Could you check a few things on this model? Use its own coordinates, in mm. Face numbers are marked on the shaded views. A direction names the side the tool comes from. Coordinates: 2 decimals unless noted, no trailing zeros. Write each loop counter-clockwise with the first axis right and the second up, starting at its lowest first coordinate (ties: lowest second). Pieces come first, ordered by that corner, then holes.
Autodesk Inventor part; units mm, degrees
ref_plane "Plano de trabajo1" through (15, 0, 0) normal (1, 0, 0) x (0, 1, 0)
ref_plane "Plano de trabajo2" through (0, 0, 7.5) normal (0, 0, 1) x (1, 0, 0)
ref_plane "XZ Plane" through (0, 0, 0) normal (0, 1, 0) x (-1, 0, 0)
sketch "Boceto1" plane through (0, 0, 0) normal (0, 1, 0) x (-1, 0, 0)
  circle A0 centre (0, 0) radius 15
  dimension "d0" = 30
extrude "Extrusión1" add sketch "Boceto1" along normal blind 10
sketch "Boceto2" plane through (0, 10, 0) normal (0, 1, 0) x (1, 0, 0)
  circle A0 centre (0, 0) radius 5
  dimension "d3" = 10
extrude "Extrusión2" cut sketch "Boceto2" against normal blind 5
sketch "Boceto3" plane through (0, 0, 0) normal (0, -1, 0) x (1, 0, 0)
  circle A0 centre (0, 0) radius 7.5
  dimension "d6" = 15
extrude "Extrusión3" add sketch "Boceto3" along normal blind 10
sketch "Boceto4" plane through (0, -10, 0) normal (0, -1, 0) x (1, 0, 0)
  circle A0 centre (0, 0) radius 2.975
  dimension "d9" = 5.95
extrude "Extrusión4" cut sketch "Boceto4" against normal blind 5
sketch "Boceto5" plane through (0, 10, 0) normal (0, 1, 0) x (1, 0, 0)
  circle A0 centre (0, 0) radius 5
  circle A1 centre (0, 0) radius 15
extrude "Extrusión5" add sketch "Boceto5" along normal blind 5
sketch "Boceto6" plane through (0, -10, 0) normal (0, -1, 0) x (1, 0, 0)
  circle A0 centre (0, 0) radius 2.975
  circle A1 centre (0, 0) radius 7.5
extrude "Extrusión6" add sketch "Boceto6" along normal blind 5
chamfer "Chaflán1" distance 1 angle 45 1 edges at (-7.5, -15, 0)
chamfer "Chaflán2" distance 1 angle 45 1 edges at (15, 0, 0)
chamfer "Chaflán3" distance 1 angle 45 1 edges at (-15, 15, 0)
fillet "Empalme1" radius 2 1 edges at (-7.5, 0, 0)
ref_plane "Plano de trabajo1" through (15, 0, 0) normal (1, 0, 0) x (0, 1, 0)
sketch "Boceto7" plane through (15, 0, 0) normal (1, 0, 0) x (0, 1, 0)
  line L0 (1, 15) -> (1, -15)
  line L1 (14, -15) -> (14, 15)
  line L2 (1, -15) -> (14, -15)
  line L3 (1, 15) -> (14, 15)
  line L4 (7.5, 15) -> (7.5, -15) construction
  circle A0 centre (7.5, 0) radius 1.5
  point P0 (0, 0)
  dimension "d27" = 3
extrude "Extrusión7" cut sketch "Boceto7" against normal blind 11 contours A0
ref_plane "Plano de trabajo2" through (0, 0, 7.5) normal (0, 0, 1) x (1, 0, 0)
sketch "Boceto8" plane through (0, 0, 7.5) normal (0, 0, 1) x (1, 0, 0)
  line L0 (-7.5, -14) -> (7.5, -14)
  line L1 (7.5, -2) -> (-7.5, -2)
  line L2 (7.5, -2) -> (7.5, -14)
  line L3 (-7.5, -2) -> (-7.5, -14)
  line L4 (7.5, -8) -> (-7.5, -8) construction
  circle A0 centre (0, -8) radius 1.5
  point P0 (0, 0)
  dimension "d31" = 3
extrude "Extrusión8" cut sketch "Boceto8" against normal blind 6 contours A0
properties part number "Acople_EJE" material "Plástico ABS"
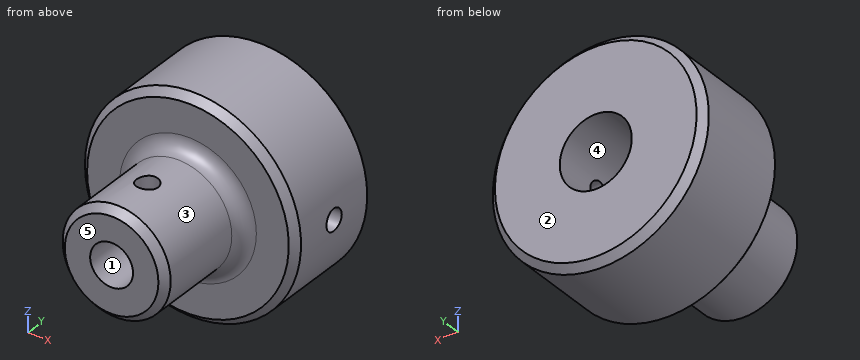
1. I want a section at A-A on y = -12. Please give me the cut outline in (x, z) (3 decimals), plus the area to 3 significant figures.
Verdict:
outline: circle Ø15 at (0, 0); hole circle Ø5.95 at (0, 0)
area: 149 mm2
2. I want a section at C-C on y = 2. Please give me the cut outline in (x, z), plus the area to 3 significant figures.
Verdict:
outline: circle Ø30 at (0, 0)
area: 707 mm2
3. For pin 1 (3 mm diameter, centred on x = -2.5, z = -2, fed in from +Y); pin 2 (2 mm diameter, centred on x = 7.5, y = 7.5, fed in from +Z); pin 3 (3 mm diameter, centred on y = -6, z = -4.5, fed in from +X), each with a flat end and sliding along its axis, tell me the tip position at first contact or that it passes through.
Verdict:
pin 1: stops at y = 5
pin 2: stops at z = 13.52
pin 3: stops at x = 6.87
4. On a 3-axis mill with a long thin cutter (end or side, diameter ignored), from which of +Z, -Z, +X, -X, +Y, -Y can I reach the whole of each face in a straight line? I mean the marked faces 1 and 2. Say none if no direction works.
Verdict:
face 1: -Y
face 2: +Z, -Z, +X, -X, +Y
5. I want a section at D-D on y = -8. Please give me the cut outline in (x, z) (3 decimals).
Verdict:
outline: (-1.5, 2.569) - (-1.5, 7.348) arc R7.5 ccw (long way) to (1.5, 7.348) - (1.5, 2.569) arc R2.975 cw (long way) to start
6. If we mould it in two halves opening along X, with no side actions, what happens to the marked faces 3, 4 and 5? For each: pulls with the +X half, pulls with the -X half, needs draft (parallel to the pull), parting line crosses it, or undercut.
Verdict:
face 3: parting line crosses it
face 4: undercut
face 5: needs draft
7. Please list where these lines run through material, in increasing order: line 1 along Y through (x, z) = (0, 5.55); line 2 along Y through (x, z) = (9.5, 0); line 3 along Z through (x, y) = (0, -11) (3 decimals).
Verdict:
line 1: y = -15 to -9.5, -6.5 to 15
line 2: y = 0 to 6, 9 to 15
line 3: z = -7.5 to -2.975, 2.975 to 7.5
